Verification items for the finished model (mm, model axes). Face numbers are marked on the shaded views. A direction names the side the tool comes from. Give positions to 0.01 mm unless a question says otherwise; leave off trailing zeros. Write each loop counter-clockwise with the first axis right and the second up, starting at its lowest first coordinate (ties: lowest second). Pieces come first, ordered by that corner, then holes.
from build123d import *

# Parameters (mm, degrees)
SKETCH6_W           = 300
SKETCH6_H           = 200
BOSS_EXTRUDE2_DEPTH = 400
SKETCH7_W           = 280
SKETCH7_H           = 190
CUT_EXTRUDE1_DEPTH  = 390
SKETCH8_R           = 52.806459668
BOSS_EXTRUDE3_DEPTH = 1000
SKETCH9_R           = 3.5
CUT_EXTRUDE3_DEPTH  = 5
CUT_EXTRUDE4_REACH  = 1113.602
SKETCH10_W          = 300
SKETCH10_H          = 10


with BuildPart() as part:
    # Sketch6 → Boss-Extrude2 (new body)
    with BuildSketch(Plane.XY):
        with Locations((125.060423937, -72.070983455)):
            Rectangle(SKETCH6_W, SKETCH6_H)
    extrude(amount=BOSS_EXTRUDE2_DEPTH)

    # Sketch7 → Cut-Extrude1 (cut)
    with BuildSketch(Plane(origin=(0, 0, 0), x_dir=(-1, 0, 0), z_dir=(0, 0, -1))):
        with Locations((-125.060423937, -72.070983455)):
            Rectangle(SKETCH7_W, SKETCH7_H)
    extrude(amount=-CUT_EXTRUDE1_DEPTH, mode=Mode.SUBTRACT)

    # Sketch8 → Boss-Extrude3 (add)
    with BuildSketch(Plane.XZ.offset(172.070983455)):
        with Locations(Location((125.060423937, 200, 0), (0, 0, 270))):
            Circle(SKETCH8_R)
    extrude(amount=BOSS_EXTRUDE3_DEPTH)

    # Sketch9 → Cut-Extrude3 (cut)
    with BuildSketch(Plane.XZ.offset(172.070983455)):
        with Locations(Location((45.060423937, 15, 0), (0, 0, 270))):
            Circle(SKETCH9_R)
        with Locations(Location((205.060423937, 15, 0), (0, 0, 270))):
            Circle(SKETCH9_R)
    extrude(amount=-CUT_EXTRUDE3_DEPTH, mode=Mode.SUBTRACT)

    # Cut-Extrude4: up to this face of the body (flat: up to its plane)
    cut_extrude4_end = Plane(part.part.faces().sort_by_distance((125.060423937, 27.929016545, 200))[0])
    # Sketch10 → Cut-Extrude4 (cut, up to the picked face)
    with BuildSketch(Plane.XZ.offset(172.070983455), mode=Mode.PRIVATE) as cut_extrude4_sk1:
        with Locations((125.060423937, 5)):
            Rectangle(SKETCH10_W, SKETCH10_H)
    cut_extrude4_tool1 = split(extrude(cut_extrude4_sk1.sketch, amount=-CUT_EXTRUDE4_REACH, mode=Mode.PRIVATE), bisect_by=cut_extrude4_end, keep=Keep.BOTH, mode=Mode.PRIVATE)
    add(cut_extrude4_tool1.solids().sort_by(Axis((125.060424, -172.070983, 5), (0, 1, 0)))[0], mode=Mode.SUBTRACT)


solid = part.part
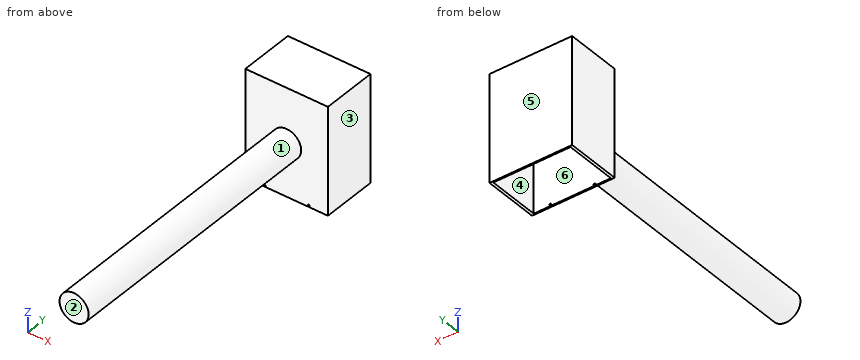
Item 1: Sectioned sample at C-C on y = -58.5. Record the cut outline in (x, z), then the cut area to 3 significant figures.
Answer key:
outline: (-24.94, 10) - (-14.94, 10) - (-14.94, 390) - (265.06, 390) - (265.06, 10) - (275.06, 10) - (275.06, 400) - (-24.94, 400) - close
area: 10,600 mm2
Item 2: Sectioned sample at D-D on x = 87. Record the cut outline in (y, z) (3 decimals).
Answer key:
outline: (-1172.071, 163.395) - (-172.071, 163.395) - (-172.071, 10) - (-167.071, 10) - (-167.071, 390) - (22.929, 390) - (22.929, 10) - (27.929, 10) - (27.929, 400) - (-172.071, 400) - (-172.071, 236.605) - (-1172.071, 236.605) - close
Item 3: Sectioned sample at A-A on x = 227. Record the cut outline in (y, z), then the cut area to 3 significant figures.
Answer key:
outline: (-172.07, 10) - (-167.07, 10) - (-167.07, 390) - (22.93, 390) - (22.93, 10) - (27.93, 10) - (27.93, 400) - (-172.07, 400) - close
area: 5,800 mm2
Item 4: Set-up check for the marked faces 1 and 2: record each of +Z, -Z, +X, -X, +Y, -Y from which the full face is reachable in a straight line by a thin tool's end or side.
Answer key:
face 1: -Y
face 2: +Z, -Z, +X, -X, -Y
Item 5: Release check for a two-part mould opening along X. For the marked faces 3, 4, 5 and 6 record: released by +X, released by -X, zero draft, split by the parting line, or undercut.
Answer key:
face 3: released by +X
face 4: undercut
face 5: zero draft
face 6: undercut
Item 6: Scan lines: line 1 along X through (y, z) = (-170, 15); line 2 along Y through (x, z) = (51.5, 151); line 3 along Y through (x, z) = (158.5, 234.5). Record each from-to range of solid material in increasing order.
Answer key:
line 1: x = -24.94 to 41.56, 48.56 to 201.56, 208.56 to 275.06
line 2: y = -172.07 to -167.07, 22.93 to 27.93
line 3: y = -1172.07 to -167.07, 22.93 to 27.93
Item 7: Sectioned sample at B-B on z = 200. Record the cut outline in (x, y), then the cut area to 3 significant figures.
Answer key:
outline: (-24.94, -172.07) - (72.25, -172.07) - (72.25, -1172.07) - (177.87, -1172.07) - (177.87, -172.07) - (275.06, -172.07) - (275.06, 27.93) - (-24.94, 27.93) - close; hole (-14.94, -167.07) - (265.06, -167.07) - (265.06, 22.93) - (-14.94, 22.93) - close
area: 112,000 mm2
Item 8: Depth check by flat-ended pin: pin 1 (1.5 mm diameter, centred on y = -923.5, z = 209, fed in from +X); pin 2 (8 mm diameter, centred on x = 45.06, z = 15, fed in from -Y); pin 3 (1 mm diameter, centred on x = 82, y = -235, fed in from +Z). Enter the tip coordinate at first touch or a pass-through.
Answer key:
pin 1: stops at x = 177.22
pin 2: stops at y = -172.07
pin 3: stops at z = 231.26
